Read the model definition and answer for the solid it produces. Units are mm, in the model's axes. Face numbers are marked on the shaded views. Give positions to 0.01 mm unless a question says otherwise; leave off trailing zeros. Order: outer loops, then holes, each group sorted by start corner. A loop starts at its lowest first (then second) coordinate and runs counter-clockwise, first axis right, second up. Notation, with made-up numbers: (-28.5, 78.25) - (10.5, 78.25) arc R9 cw to (10.5, 83.25) - close; hole circle Ø10 at (-34.75, 44.5). An arc over 180 degrees is marked (long way). Write each question's results on one line, items separated by ' | '.
from build123d import *

# Parameters (mm, degrees)
SKETCH1_W           = 50
SKETCH1_H           = 20
BOSS_EXTRUDE1_DEPTH = 6
SKETCH1_3_R         = 2.5
SKETCH1_3_R_2       = 1.5
CUT_EXTRUDE1_DEPTH  = 6


with BuildPart() as part:
    # Sketch1 → Boss-Extrude1 (new body)
    with BuildSketch(Plane(origin=(0, 0, 0), x_dir=(1, 0, 0), z_dir=(0, 1, 0))):
        Rectangle(SKETCH1_W, SKETCH1_H)
    extrude(amount=BOSS_EXTRUDE1_DEPTH)

    # Sketch1<3> → Cut-Extrude1 (cut)
    with BuildSketch(Plane(origin=(0, 0, 0), x_dir=(1, 0, 0), z_dir=(0, 1, 0))):
        with Locations((20, 0)):
            Circle(SKETCH1_3_R)
        with Locations((-10, 0)):
            Circle(SKETCH1_3_R)
        with Locations((10, 0)):
            Circle(SKETCH1_3_R)
        with Locations((-22.5, 0)):
            Circle(SKETCH1_3_R_2)
    extrude(amount=CUT_EXTRUDE1_DEPTH, mode=Mode.SUBTRACT)


solid = part.part
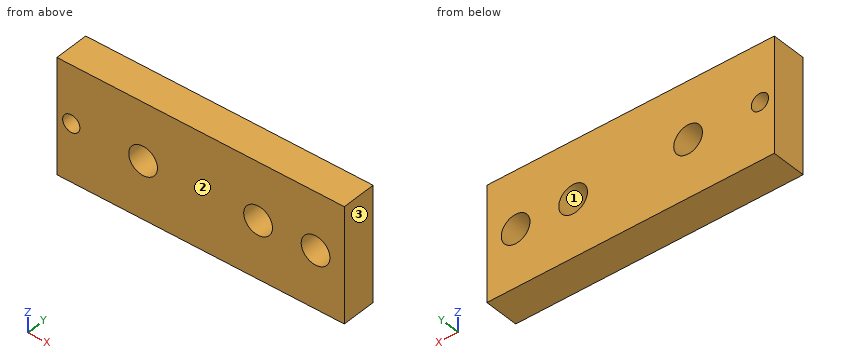
(1) Consider probe 1 along X at (y, z) = (3.3, 0); probe 2 along X at (y, z) = (4.7, -2); probe 3 along Z at (x, y) = (-22.5, 4). Determine where each line is inside the solid, lowest interval first. Write a range as [from, to].
Conclusion:
probe 1: [-25, -24], [-21, -12.5], [-7.5, 7.5], [12.5, 17.5], [22.5, 25] | probe 2: [-25, -11.5], [-8.5, 8.5], [11.5, 18.5], [21.5, 25] | probe 3: [-10, -1.5], [1.5, 10]
(2) Section C-C (y = 0.5) is taken. Give the vertices of the cut face in (x, z).
Conclusion:
outline: (-25, -10) - (25, -10) - (25, 10) - (-25, 10) - close; hole circle Ø3 at (-22.5, 0); hole circle Ø5 at (-10, 0); hole circle Ø5 at (10, 0); hole circle Ø5 at (20, 0)
(3) Section D-D (x = -22.5) is taken. Give the vertices of the cut face in (y, z).
Conclusion:
outline: (0, -10) - (6, -10) - (6, -1.5) - (0, -1.5) - close; (0, 1.5) - (6, 1.5) - (6, 10) - (0, 10) - close
(4) This flat-tipped pin is pushed along its axis until it touches: pin 1 (6 mm diameter, centred on x = -10, z = 0, fed in from -Y). Where does it stop, or does it pass through?
Conclusion:
pin 1: y = 0
(5) The mould has two halves that part along X. Classify the marked faces 1, 2 and 3: pulls with the +X half, pulls with the -X half, needs draft (parallel to the pull), parting line crosses it, or undercut.
Conclusion:
face 1: undercut | face 2: needs draft | face 3: pulls with the +X half
(6) Section B-B (x = -10) is taken. Give the vertices of the cut face in (y, z).
Conclusion:
outline: (0, -10) - (6, -10) - (6, -2.5) - (0, -2.5) - close; (0, 2.5) - (6, 2.5) - (6, 10) - (0, 10) - close
(7) Section A-A (z = 0) is taken. Give the vertices of the cut face in (x, y), plus the area to 3 significant figures.
Conclusion:
outline: (-25, 0) - (-24, 0) - (-24, 6) - (-25, 6) - close; (-21, 0) - (-12.5, 0) - (-12.5, 6) - (-21, 6) - close; (-7.5, 0) - (7.5, 0) - (7.5, 6) - (-7.5, 6) - close; (12.5, 0) - (17.5, 0) - (17.5, 6) - (12.5, 6) - close; (22.5, 0) - (25, 0) - (25, 6) - (22.5, 6) - close | area: 192 mm^2
